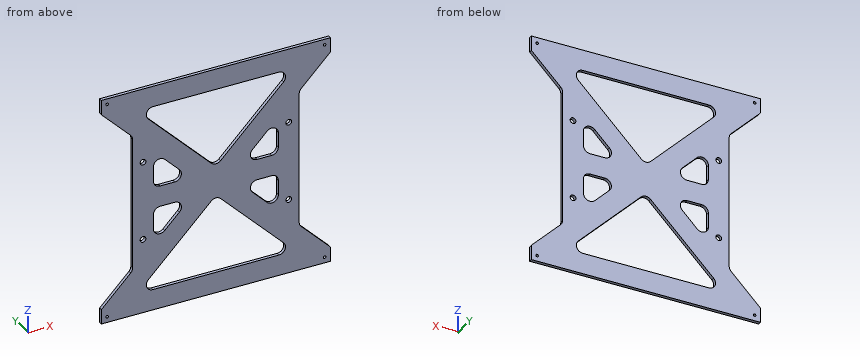
```python
from build123d import *

# Parameters (mm, degrees)
SKETCH1_W             = 220
SKETCH1_H             = 220
BOSS_EXTRUDE1_DEPTH   = 3.175
M3X0_5_TAPPED_HOLE1_D = 2.5
SKETCH4_R             = 2.75
CUT_EXTRUDE1_DEPTH    = 4.175
CUT_EXTRUDE2_DEPTH    = 4.175


with BuildPart() as part:
    # Sketch1 → Boss-Extrude1 (new body)
    with BuildSketch(Plane(origin=(0, 0, 0), x_dir=(1, 0, 0), z_dir=(0, 1, 0))):
        Rectangle(SKETCH1_W, SKETCH1_H)
    extrude(amount=BOSS_EXTRUDE1_DEPTH)

    # M3x0.5 Tapped Hole1 (through all)
    with Locations(Plane(origin=(0, 3.175, 0), x_dir=(-1, 0, 0), z_dir=(0, 1, 0))):
        with Locations((104.5, -104.5), (-104.5, -104.5), (-104.5, 104.5), (104.5, 104.5)):
            Hole(M3X0_5_TAPPED_HOLE1_D / 2)

    # Sketch4 → Cut-Extrude1 (cut, through all)
    with BuildSketch(Plane(origin=(0, 3.175, 0), x_dir=(1, 0, 0), z_dir=(0, 1, 0))):
        with Locations(Location((-70, 38, 0), (0, 0, 270))):  # turned: the seam where the file's is
            Circle(SKETCH4_R)
        with Locations(Location((-70, -38, 0), (0, 0, 270))):  # turned: the seam where the file's is
            Circle(SKETCH4_R)
        with Locations(Location((70, -38, 0), (0, 0, 270))):  # turned: the seam where the file's is
            Circle(SKETCH4_R)
        with Locations(Location((70, 38, 0), (0, 0, 270))):  # turned: the seam where the file's is
            Circle(SKETCH4_R)
    extrude(amount=-CUT_EXTRUDE1_DEPTH, mode=Mode.SUBTRACT)

    # Sketch5 → Cut-Extrude2 (cut, through all)
    with BuildSketch(Plane(origin=(0, 3.175, 0), x_dir=(1, 0, 0), z_dir=(0, 1, 0))):
        with BuildLine():
            Line((-65.017736316, 79.159871939), (-4.490128061, 18.632263684))
            ThreePointArc((-4.490128061, 18.632263684), (0, 16.772391745), (4.490128061, 18.632263684))
            Line((4.490128061, 18.632263684), (65.017736316, 79.159871939))
            ThreePointArc((65.017736316, 79.159871939), (66.394243287, 86.080039796), (60.527608255, 90))
            Line((60.527608255, 90), (-60.527608255, 90))
            ThreePointArc((-60.527608255, 90), (-66.394243287, 86.080039796), (-65.017736316, 79.159871939))
        make_face()
        with BuildLine():
            Line((-4.490128061, -18.632263684), (-65.017736316, -79.159871939))
            ThreePointArc((-65.017736316, -79.159871939), (-66.394243287, -86.080039796), (-60.527608255, -90))
            Line((-60.527608255, -90), (60.527608255, -90))
            ThreePointArc((60.527608255, -90), (66.394243287, -86.080039796), (65.017736316, -79.159871939))
            Line((65.017736316, -79.159871939), (4.490128061, -18.632263684))
            ThreePointArc((4.490128061, -18.632263684), (0, -16.772391745), (-4.490128061, -18.632263684))
        make_face()
        with BuildLine():
            Line((-60, -16.35), (-60, -30.527608255))
            ThreePointArc((-60, -30.527608255), (-56.080039796, -36.394243287), (-49.159871939, -35.017736316))
            Line((-49.159871939, -35.017736316), (-34.982263684, -20.840128061))
            ThreePointArc((-34.982263684, -20.840128061), (-33.605756713, -13.919960204), (-39.472391745, -10))
            Line((-39.472391745, -10), (-53.65, -10))
            ThreePointArc((-53.65, -10), (-58.140128061, -11.859871939), (-60, -16.35))
        make_face()
        with BuildLine():
            Line((39.472391745, -10), (53.65, -10))
            ThreePointArc((53.65, -10), (58.140128061, -11.859871939), (60, -16.35))
            Line((60, -16.35), (60, -30.527608255))
            ThreePointArc((60, -30.527608255), (56.080039796, -36.394243287), (49.159871939, -35.017736316))
            Line((49.159871939, -35.017736316), (34.982263684, -20.840128061))
            ThreePointArc((34.982263684, -20.840128061), (33.605756713, -13.919960204), (39.472391745, -10))
        make_face()
        with BuildLine():
            Line((34.982263684, 20.840128061), (49.159871939, 35.017736316))
            ThreePointArc((49.159871939, 35.017736316), (56.080039796, 36.394243287), (60, 30.527608255))
            Line((60, 30.527608255), (60, 16.35))
            ThreePointArc((60, 16.35), (58.140128061, 11.859871939), (53.65, 10))
            Line((53.65, 10), (39.472391745, 10))
            ThreePointArc((39.472391745, 10), (33.605756713, 13.919960204), (34.982263684, 20.840128061))
        make_face()
        with BuildLine():
            Line((-39.472391745, 10), (-53.65, 10))
            ThreePointArc((-53.65, 10), (-58.140128061, 11.859871939), (-60, 16.35))
            Line((-60, 16.35), (-60, 30.527608255))
            ThreePointArc((-60, 30.527608255), (-56.080039796, 36.394243287), (-49.159871939, 35.017736316))
            Line((-49.159871939, 35.017736316), (-34.982263684, 20.840128061))
            ThreePointArc((-34.982263684, 20.840128061), (-33.605756713, 13.919960204), (-39.472391745, 10))
        make_face()
        with BuildLine():
            Line((-110, 95.857864376), (-110, -95.857864376))
            Line((-110, -95.857864376), (-81.859871939, -67.717736316))
            ThreePointArc((-81.859871939, -67.717736316), (-80.483364969, -65.657648051), (-80, -63.227608255))
            Line((-80, -63.227608255), (-80, 63.227608255))
            ThreePointArc((-80, 63.227608255), (-80.483364969, 65.657648051), (-81.859871939, 67.717736316))
            Line((-81.859871939, 67.717736316), (-110, 95.857864376))
        make_face()
        with BuildLine():
            Line((110, 95.857864376), (81.859871939, 67.717736316))
            ThreePointArc((81.859871939, 67.717736316), (80.483364969, 65.657648051), (80, 63.227608255))
            Line((80, 63.227608255), (80, -63.227608255))
            ThreePointArc((80, -63.227608255), (80.483364969, -65.657648051), (81.859871939, -67.717736316))
            Line((81.859871939, -67.717736316), (110, -95.857864376))
            Line((110, -95.857864376), (110, 95.857864376))
        make_face()
    extrude(amount=-CUT_EXTRUDE2_DEPTH, mode=Mode.SUBTRACT)


solid = part.part
```
Source: CAD feature listing. Evaluate the final solid. Frame: model axes, mm. Coordinates: 2 decimals unless noted, no trailing zeros. Loops run counter-clockwise (first coordinate to the right, second up) from the corner with the lowest first, then second, coordinate; pieces in that order, holes last. Notation, with made-up numbers: M -29,12 L -14,12 A28 ccw -14,48 Z; hole C -18.5,18.25 d4. An arc over 180 degrees is marked long. Use a Markdown table: item, result. Add a question column.
Q1. Section query B-B, the plane x = 85. Return loops of the section in (y, z) (3 decimals), and give its area (3 significant figures).
Q2. Material intervals for L1, parallel to X at y = 2.4, z = -104.5; L2, parallel to Z at x = 104.5, y = 0.7; L3, parallel to Z at x = 52, y = 0.55, sorted ascending.
Q3. Section query D-D, the plane z = -5.5. Return loops of the section in (x, y) (3 decimals).
Q4. Section query A-A, the plane x = -70. Return loops of the section in (y, z) (3 decimals), and give its area (3 significant figures).
Q5. First-contact query: pin 1 (1.5 mm diameter, centred on x = -74, z = -26.5, fed in from -Y); pin 2 (1 mm diameter, centred on y = 2, z = 22, fed in from -X); pin 3 (3.5 mm diameter, centred on x = 70, z = 38, fed in from -Y); pin 4 (1 mm diameter, centred on y = 2, z = 16, fed in from +X). Flat tips, straight axial feed; report the tip coordinate or a pass-through.
Q6. Section query C-C, the plane y = 1.25. State how many separate pieces and enclosed holes the cut face has, and give its area (3 significant figures).
Result:
| question | item | result |
|---|---|---|
| 1 | outline | M 0,-110 L 3.175,-110 L 3.175,-70.858 L 0,-70.858 Z; M 0,70.858 L 3.175,70.858 L 3.175,110 L 0,110 Z |
| 1 | area | 249 mm2 |
| 2 | L1 | x = -110 to -105.75, -103.25 to 103.25, 105.75 to 110 |
| 2 | L2 | z = -110 to -105.75, -103.25 to -90.36, 90.36 to 103.25, 105.75 to 110 |
| 2 | L3 | z = -110 to -90, -66.14 to -36.66, -10 to 10, 36.66 to 66.14, 90 to 110 |
| 3 | outline | M -80,0 L 80,0 L 80,3.175 L -80,3.175 Z |
| 4 | outline | M 0,-110 L 3.175,-110 L 3.175,-40.75 L 0,-40.75 Z; M 0,-35.25 L 3.175,-35.25 L 3.175,35.25 L 0,35.25 Z; M 0,40.75 L 3.175,40.75 L 3.175,110 L 0,110 Z |
| 4 | area | 664 mm2 |
| 5 | pin 1 | stops at y = 0 |
| 5 | pin 2 | stops at x = -80 |
| 5 | pin 3 | passes through |
| 5 | pin 4 | stops at x = 80 |
| 6 | separate pieces | 1 |
| 6 | enclosed holes | 14 |
| 6 | area | 25,200 mm2 |
